The listing builds one solid part. Answer for the finished solid, in the listing's coordinates (mm). A direction names the side the tool comes from. Round coordinates to 2 decimals unless told otherwise and drop trailing zeros. Loops run counter-clockwise (first coordinate to the right, second up) from the corner with the lowest first, then second, coordinate; pieces in that order, holes last. Notation, with made-up numbers: (48.5, 30.25) -> (94.5, 30.25) arc R28 ccw to (94.5, 56.25) -> close; hole circle Ø8 at (76.25, 40). An arc over 180 degrees is marked (long way). Use a Markdown table: item, result. Add a question column.
Q1. For a pull along Z with two mould halves and no side action, classify faces 1 (the cylindrical face through (18.88, 2.5, -22.27)), 2 (the flat face through (89, 3, -127)), 3 (the flat face through (33, 9, -2.832)) as released by +Z, released by -Z, zero draft, split by the parting line, or undercut.
Q2. Section C-C on x = 150 is taken. Give the vertices of the cut face in (y, z).
Q3. Which of the six approach directions +Z, -Z, +X, -X, +Y, -Y give full straight-line access (tool end or side, diameter ignored) to faces 4 (the flat face through (89, 9, -124.168)), 5 (the flat face through (82, 9, -84.62)), 6 (the flat face through (173.99, 9, -63)), 7 (the flat face through (175.768, 9, -64)), 8 (the flat face through (89, 0, -64))?
Q4. Given pin 1 Ø4 at (x, y) = (70, 9.5) entering from +Z; pin 2 Ø5 at (x, y) = (127, 6) entering from -Z; pin 3 Ø6 at (y, z) = (9.5, -78.5) entering from +X; pin 4 Ø5 at (x, z) = (149.5, -23.5) entering from +Y, each flat-ended and moving along its own axis, determine where each tip first touches the part or whether it passes through.
Q5. Consider line 1 (X direction, y = 5.25, z = -7.5); line 2 (Z direction, x = 77, y = 11.25); line 3 (Z direction, x = 48.26, y = 3.5). Determine where each line is inside the solid, lowest interval first.
Q6. Section B-B on z = -113.5 is taken. Give the vertices of the cut face in (x, y).
Q7. Section D-D on z = -54 is taken. Give the vertices of the cut face in (x, y).
Q8. Section A-A on x = 30.26 is taken. Give the vertices of the cut face in (y, z).
from build123d import *

# Parameters (mm, degrees)
SKETCH1_W           = 180.34
SKETCH1_H           = 127
BOSS_EXTRUDE1_DEPTH = 5.08
BOSS_EXTRUDE2_DEPTH = 7.62
SKETCH3_R           = 3
CUT_EXTRUDE1_DEPTH  = 10.16


with BuildPart() as part:
    # Sketch1 → Boss-Extrude1 (new body)
    with BuildSketch(Plane(origin=(0, 0, 0), x_dir=(1, 0, 0), z_dir=(0, 1, 0))):
        with Locations((90.17, 63.5)):
            Rectangle(SKETCH1_W, SKETCH1_H)
    extrude(amount=BOSS_EXTRUDE1_DEPTH)

    # Sketch2 → Boss-Extrude2 (add)
    with BuildSketch(Plane(origin=(0, 5.08, 0), x_dir=(1, 0, 0), z_dir=(0, 1, 0))):
        Polygon((4.572, 124.1679), (175.768, 124.1679), (175.768, 2.8321), (103.4542, 2.8321), (103.4542, 84.6201), (59.69, 84.6201), (59.69, 2.8321), (4.572, 2.8321), align=None)
        Polygon((6.35, 122.3899), (6.35, 4.6101), (57.912, 4.6101), (57.912, 86.3981), (105.2322, 86.3981), (105.2322, 4.6101), (173.99, 4.6101), (173.99, 122.3899), align=None, mode=Mode.SUBTRACT)
    extrude(amount=BOSS_EXTRUDE2_DEPTH)

    # Sketch3 → Cut-Extrude1 (cut)
    with BuildSketch(Plane.XZ):
        with Locations((21.26, -20.440905976)):
            Circle(SKETCH3_R)
        with Locations((30.26, -20.440905976)):
            Circle(SKETCH3_R)
        with Locations((39.26, -20.440905976)):
            Circle(SKETCH3_R)
        with Locations((48.26, -20.440905976)):
            Circle(SKETCH3_R)
    extrude(amount=-CUT_EXTRUDE1_DEPTH, mode=Mode.SUBTRACT)


solid = part.part
Checked values:
| question | item | result |
|---|---|---|
| 1 | face 1 | undercut |
| 1 | face 2 | released by -Z |
| 1 | face 3 | released by +Z |
| 2 | outline | (0, -127) -> (5.08, -127) -> (5.08, -124.17) -> (12.7, -124.17) -> (12.7, -122.39) -> (5.08, -122.39) -> (5.08, -4.61) -> (12.7, -4.61) -> (12.7, -2.83) -> (5.08, -2.83) -> (5.08, 0) -> (0, 0) -> close |
| 3 | face 4 | -Z, +X, -X, +Y |
| 3 | face 5 | +Z, +Y |
| 3 | face 6 | +Y |
| 3 | face 7 | +Z, -Z, +X, +Y |
| 3 | face 8 | +Z, -Z, +X, -X, -Y |
| 4 | pin 1 | stops at z = -84.62 |
| 4 | pin 2 | stops at z = -127 |
| 4 | pin 3 | stops at x = 175.77 |
| 4 | pin 4 | stops at y = 5.08 |
| 5 | line 1 | x = 4.57 to 6.35, 57.91 to 59.69, 103.45 to 105.23, 173.99 to 175.77 |
| 5 | line 2 | z = -124.17 to -122.39, -86.4 to -84.62 |
| 5 | line 3 | z = -127 to -23.44, -17.44 to 0 |
| 6 | outline | (0, 0) -> (180.34, 0) -> (180.34, 5.08) -> (175.77, 5.08) -> (175.77, 12.7) -> (173.99, 12.7) -> (173.99, 5.08) -> (6.35, 5.08) -> (6.35, 12.7) -> (4.57, 12.7) -> (4.57, 5.08) -> (0, 5.08) -> close |
| 7 | outline | (0, 0) -> (180.34, 0) -> (180.34, 5.08) -> (175.77, 5.08) -> (175.77, 12.7) -> (173.99, 12.7) -> (173.99, 5.08) -> (105.23, 5.08) -> (105.23, 12.7) -> (103.45, 12.7) -> (103.45, 5.08) -> (59.69, 5.08) -> (59.69, 12.7) -> (57.91, 12.7) -> (57.91, 5.08) -> (6.35, 5.08) -> (6.35, 12.7) -> (4.57, 12.7) -> (4.57, 5.08) -> (0, 5.08) -> close |
| 8 | outline | (0, -127) -> (5.08, -127) -> (5.08, -124.17) -> (12.7, -124.17) -> (12.7, -122.39) -> (5.08, -122.39) -> (5.08, -23.44) -> (0, -23.44) -> close; (0, -17.44) -> (5.08, -17.44) -> (5.08, -4.61) -> (12.7, -4.61) -> (12.7, -2.83) -> (5.08, -2.83) -> (5.08, 0) -> (0, 0) -> close |
